Autodesk Inventor part; units mm, degrees
ref_plane "YZ Plane" through (0, 0, 0) normal (1, 0, 0) x (0, 1, 0)
ref_plane "XZ Plane" through (0, 0, 0) normal (0, 1, 0) x (-1, 0, 0)
ref_plane "XY Plane" through (0, 0, 0) normal (0, 0, 1) x (1, 0, 0)
sketch "Sketch4" plane through (0, 0, 0) normal (0, 1, 0) x (-1, 0, 0)
  circle A0 centre (0, 0) radius 39.75
  circle A1 centre (0, 0) radius 41.6215
  circle A2 centre (0, 0) radius 41.6213
  dimension "d17" = 79.5
  dimension "d18" = 83.243
sketch "Sketch6" plane through (0, 0, 0) normal (0, 1, 0) x (-1, 0, 0)
  circle A0 centre (0, 0) radius 39.7618
extrude "Extrusion1" add sketch "Sketch6" along normal blind 3
extrude "Extrusion2" add sketch "Sketch4" along normal blind 9
sketch "Sketch7" plane through (0, 0, 0) normal (0, -1, 0) x (1, 0, 0)
  circle A0 centre (0, 0) radius 44.86
  circle A1 centre (0, 0) radius 41.6213
extrude "Extrusion3" add sketch "Sketch7" against normal blind 14
sketch "Sketch8" plane through (0, 0, 0) normal (0, -1, 0) x (1, 0, 0)
  circle A0 centre (0, 0) radius 44.86
extrude "Extrusion4" add sketch "Sketch8" along normal blind 1
properties part number "Soft Coating Gripper mold_6mil"
Input: part model. Units: mm. Frame: model coordinates. A direction names the side the tool comes from. Round coordinates to 2 decimals unless told otherwise and drop trailing zeros. Loops run counter-clockwise (first coordinate to the right, second up) from the corner with the lowest first, then second, coordinate; pieces in that order, holes last.
1) Section query B-B on x = 0. Return the cut outline in (y, z).
Ans:
outline: (-1, -44.86) - (14, -44.86) - (14, -41.62) - (9, -41.62) - (9, -39.75) - (3, -39.75) - (3, 39.75) - (9, 39.75) - (9, 41.62) - (14, 41.62) - (14, 44.86) - (-1, 44.86) - close
2) Section query D-D on y = 6.25. Return the cut outline in (x, z), plus the area to 3 significant figures.
Ans:
outline: circle Ø89.72 at (0, 0); hole circle Ø79.5 at (0, 0)
area: 1,360 mm2
3) Section query A-A on z = 28. Return the cut outline in (x, y) (3 decimals).
Ans:
outline: (-35.049, -1) - (35.049, -1) - (35.049, 14) - (30.795, 14) - (30.795, 9) - (28.215, 9) - (28.215, 3) - (-28.215, 3) - (-28.215, 9) - (-30.795, 9) - (-30.795, 14) - (-35.049, 14) - close
4) Pull-direction query (X, two-part tool) for faces 1 (the flat face through (13, 14, -40)), 2 (the cylindrical face through (24.116, 6.395, 37.826)), 3 (the flat face through (-37, 9, -15)); classes: released by +X, released by -X, zero draft, split by the parting line, or undercut.
Ans:
face 1: zero draft
face 2: split by the parting line
face 3: undercut
5) Section query C-C on y = 0.75. Return the cut outline in (x, z).
Ans:
outline: circle Ø89.72 at (0, 0)
6) Set-up query: faces 4 (the cylindrical face through (5.175, 5.958, -39.412)), 5 (the flat face through (-1, -1, 1)). Return all of +Z, -Z, +X, -X, +Y, -Y with unobstructed straight access to the full face (end or side cutting, diameter ignored); none if empty.
Ans:
face 4: +Y
face 5: +Z, -Z, +X, -X, -Y
7) Pin query (flat end, axial travel): pin 1 (4 mm diameter, centred on x = -22.5, z = -30.5, fed in from +Y); pin 2 (2 mm diameter, centred on x = -26, y = 11.5, fed in from -Z); pin 3 (4 mm diameter, centred on y = 0.5, z = -25, fed in from -X). Return the tip coordinate at first contact, or that it passes through.
Ans:
pin 1: stops at y = 9
pin 2: stops at z = -37.25
pin 3: stops at x = -38.52
8) Material intervals for line 1 (Z direction, x = 0, y = 11.65); line 2 (Y direction, x = -12.5, z = -0.5); line 3 (X direction, y = 11.25, z = -15), sorted ascending.
Ans:
line 1: z = -44.86 to -41.62, 41.62 to 44.86
line 2: y = -1 to 3
line 3: x = -42.28 to -38.82, 38.82 to 42.28
